The model under review builds one solid part; all positions refer to its coordinate system, in mm. Coordinates: 2 decimals unless noted, no trailing zeros. Write each loop counter-clockwise with the first axis right and the second up, starting at its lowest first coordinate (ties: lowest second). Pieces come first, ordered by that corner, then holes. Notation, with made-up numbers: (37.25, -24) - (62.25, -24) arc R19 ccw to (62.25, -19) - close; hole circle Ø9 at (35, -37). An arc over 180 degrees is marked (long way). Return JSON: item names as keys, results as strings. Group by question number.
(1) We need section A-A on y = -132. State the section outline as (x, z) points, then the cut area to 3 significant figures.
(2) For pin 1 Ø4 at (x, y) = (37, -30) entering from +Z; pin 2 Ø5 at (x, y) = (60, -107.5) entering from +Z; pin 3 Ø4 at (y, z) = (-107.5, -11.5) entering from -X, all flat-tipped, find the tip position at first contact; note any pin that passes through.
(3) We need section C-C on z = -118.5. State the section outline as (x, y) points, then the cut area to 3 significant figures.
(4) To check wall thickness, follow L1, parallel to Z at x = -136.5, y = -149; L2, parallel to Z at x = -104.5, y = -46; L3, parallel to X at y = -130.5, z = 67. State the ranges of each line that lie inside material, in increasing order. Write a range as from..to.
(5) We need section B-B on x = -105. State the section outline as (y, z) points, then the cut area to 3 significant figures.
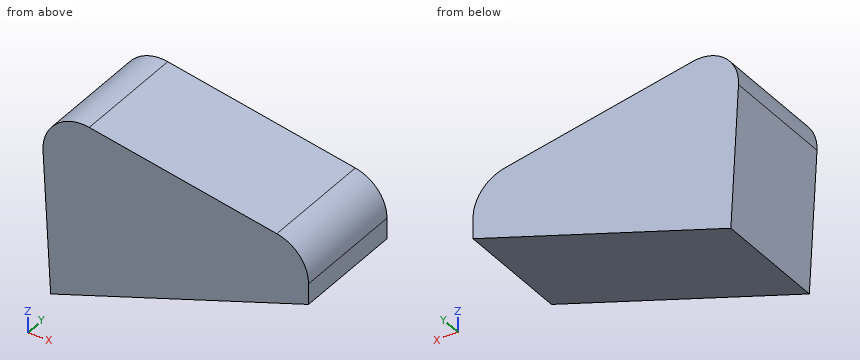
```python
from build123d import *

# Parameters (mm, degrees)
F1_DEPTH = 228.6
F2_R     = 76.2


with BuildPart() as f1:
    # F0 (on Front) → F1 (new body)
    with BuildSketch(Plane.XZ):
        Polygon((264.477155, 88.079405), (-259.452972, 188.143295), (-239.215332, -185.128794), (264.477155, -15.357443), align=None)
    extrude(amount=F1_DEPTH)

    # F2
    f2_edges = [f1.edges().sort_by_distance(p)[0] for p in [
        (-259.452972, -114.3, 188.143295),
        (264.477155, -114.3, 88.079405),
    ]]
    fillet(f2_edges, radius=F2_R)


solid = f1.part
```
Ans:
{
 "1": {"outline": "(-254.18, 90.9) - (-239.22, -185.13) - (264.48, -15.36) - (264.48, 25.06) arc R76.2 ccw to (202.57, 99.9) - (-163.8, 169.87) arc R76.2 ccw to start", "area": "120,000 mm²"},
 "2": {"pin 1": "z = 131.91", "pin 2": "z = 127.61", "pin 3": "x = -248.74"},
 "3": {"outline": "(-242.83, -228.6) - (-41.54, -228.6) - (-41.54, 0) - (-242.83, 0) - close", "area": "46,000 mm²"},
 "4": {"L1": "-150.51..164.66", "L2": "-139.72..158.55", "L3": "-252.88..251.89"},
 "5": {"outline": "(-228.6, -139.89) - (0, -139.89) - (0, 158.64) - (-228.6, 158.64) - close", "area": "68,200 mm²"}
}
